Autodesk Inventor part; units mm, degrees
ref_plane "Work Plane1" through (0, 14, 0) normal (0, 1, 0) x (1, 0, 0)
ref_plane "YZ Plane" through (0, 0, 0) normal (1, 0, 0) x (0, 1, 0)
ref_plane "XZ Plane" through (0, 0, 0) normal (0, 1, 0) x (-1, 0, 0)
sketch "Sketch1" plane through (0, 0, 0) normal (0, 1, 0) x (-1, 0, 0)
  line L0 (0, 0) -> (600, 0)
  line L1 (600, 0) -> (600, -1000)
  line L2 (600, -1000) -> (0, -1000)
  line L3 (0, -1000) -> (0, 0)
  dimension "d0" = 1000
  dimension "d1" = 600
extrude "Extrusion1" add sketch "Sketch1" along normal blind 28
sketch "Sketch2" plane through (0, 28, 0) normal (0, 1, 0) x (1, 0, 0)
  line L0 (-600, 1000) -> (-600, 0)
  line L1 (0, 1000) -> (-600, 1000)
  line L2 (0, 1000) -> (-600, 1000)
  line L3 (-600, 1000) -> (-600, 0)
  line L4 (-600, 0) -> (0, 0)
  line L5 (0, 0) -> (0, 1000)
  line L6 (-600, 100) -> (-300, 1000)
  dimension "d7" = 300
  dimension "d8" = 100
extrude "Extrusion2" cut sketch "Sketch2" against normal blind 200 contours L1 L6 L0
ref_plane "Work Plane1" through (0, 14, 0) normal (0, 1, 0) x (1, 0, 0)
sketch "Sketch3" plane through (0, 28, 0) normal (0, 1, 0) x (1, 0, 0)
  circle A0 centre (-305, 20) radius 8
  line L0 (0, 0) -> (0, 1000)
  line L1 (-600, 0) -> (0, 0)
  circle A1 centre (-395, 20) radius 8
  circle A2 centre (-350, 75) radius 8
  circle A3 centre (-350, 160) radius 8
  dimension "d9" = 16
  dimension "d10" = 305
  dimension "d11" = 20
  dimension "d12" = 16
  dimension "d13" = 395
  dimension "d14" = 20
  dimension "d15" = 16
  dimension "d16" = 350
  dimension "d17" = 75
  dimension "d18" = 16
  dimension "d19" = 350
  dimension "d20" = 160
extrude "Extrusion3" [suppressed]
chamfer "Chamfer1" distance 20 distance2 10 1 edges at (0, 28, -500) measured on face at (-300, 28, -366.6667)
chamfer "Chamfer2" distance 10 distance2 20 1 edges at (0, 0, -500) measured on face at (0, 6, -333.3333)
chamfer "Chamfer3" distance 20 distance2 10 1 edges at (-450, 28, -550) measured on face at (-306.6667, 28, -366.6667)
chamfer "Chamfer4" distance 20 distance2 10 1 edges at (-450, 0, -550) measured on face at (-306.6667, 0, -366.6667)
properties part number "Foam_wing"
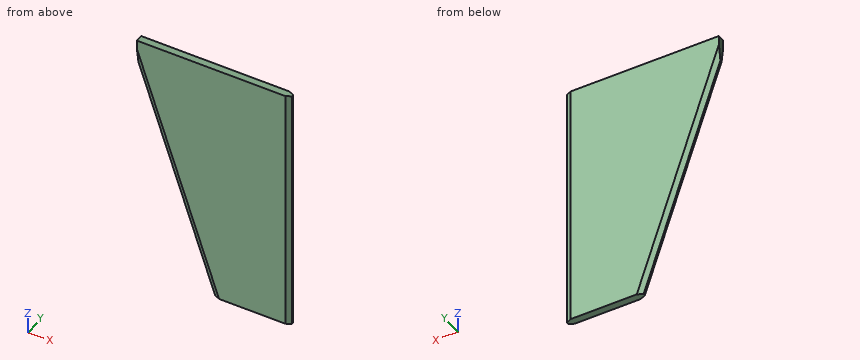
Could you check a few things on this model? Use its own coordinates, in mm. Round coordinates to 2 decimals unless told otherwise and drop trailing zeros. Loops run counter-clockwise (first coordinate to the right, second up) from the corner with the lowest first, then second, coordinate; pieces in that order, holes last. Notation, with made-up numbers: (75, 65) -> (124, 65) arc R34 cw to (124, 100) -> close; hole circle Ø2 at (60.5, 49). An arc over 180 degrees is marked (long way). Use CSV: the item, a comma, the result in double quotes.
(1) Will this pin go through, and if not, where does the flat tip stop? pin 1 Ø1 at (y, z) = (19, -288) entering from +X.
Return value:
pin 1,"stops at x = -1"
(2) Suppose I cut it at D-D on x = -321.5. Write out the boundary of the cut face in (y, z), plus the area to 3 significant figures.
Return value:
outline,"(0, -872.25) -> (10, -935.5) -> (18, -935.5) -> (28, -872.25) -> (28, 0) -> (0, 0) -> close"
area,"25,600 mm²"
(3) Suppose I cut it at B-B on x = -492.5. Write out the boundary of the cut face in (y, z).
Return value:
outline,"(0, -359.25) -> (10, -422.5) -> (18, -422.5) -> (28, -359.25) -> (28, 0) -> (0, 0) -> close"
(4) Suppose I cut it at A-A on z = -508.5. Write out the boundary of the cut face in (x, y), plus the area to 3 significant figures.
Return value:
outline,"(-463.83, 10) -> (-442.75, 0) -> (-20, 0) -> (0, 10) -> (0, 18) -> (-20, 28) -> (-442.75, 28) -> (-463.83, 18) -> close"
area,"12,600 mm²"
(5) If I drill on probe 1 along X at (y, z) = (7, -99.5); probe 2 along X at (y, z) = (15.25, -105), over which ranges is the centre line in solid material (lowest first)? Write a range as [from, to].
Return value:
probe 1,"x = [-593.84, -6]"
probe 2,"x = [-598.33, 0]"
(6) Suppose I cut it at C-C on z = -351. Write out the boundary of the cut face in (x, y), plus the area to 3 significant figures.
Return value:
outline,"(-516.33, 10) -> (-495.25, 0) -> (-20, 0) -> (0, 10) -> (0, 18) -> (-20, 28) -> (-495.25, 28) -> (-516.33, 18) -> close"
area,"14,000 mm²"
